```python
from build123d import *

# Parameters (mm, degrees)
SKETCH1_R           = 15.6
SKETCH1_R_2         = 14.3
BOSS_EXTRUDE1_DEPTH = 22
SKETCH2_R           = 18.1
SKETCH2_R_2         = 14.3
BOSS_EXTRUDE2_DEPTH = 3.5
FILLET1_R           = 1
CUT_EXTRUDE1_DEPTH  = 26.5


with BuildPart() as part:
    # Sketch1 → Boss-Extrude1 (new body)
    with BuildSketch(Plane(origin=(0, 0, 0), x_dir=(1, 0, 0), z_dir=(0, 1, 0))):
        Circle(SKETCH1_R)
        Circle(SKETCH1_R_2, mode=Mode.SUBTRACT)
    extrude(amount=BOSS_EXTRUDE1_DEPTH)

    # Sketch2 → Boss-Extrude2 (add)
    with BuildSketch(Plane(origin=(0, 22, 0), x_dir=(1, 0, 0), z_dir=(0, 1, 0))):
        Circle(SKETCH2_R)
        Circle(SKETCH2_R_2, mode=Mode.SUBTRACT)
    extrude(amount=BOSS_EXTRUDE2_DEPTH)

    # Fillet1
    fillet1_edges = [part.edges().sort_by_distance(p)[0] for p in [
        (-15.6, 22, 0),
    ]]
    fillet(fillet1_edges, radius=FILLET1_R)

    # Sketch3 → Cut-Extrude1 (cut, through all)
    with BuildSketch(Plane(origin=(0, 25.5, 0), x_dir=(1, 0, 0), z_dir=(0, 1, 0))):
        Polygon((0, 0), (-1.75, -18.1), (1.75, -18.1), align=None)
    extrude(amount=-CUT_EXTRUDE1_DEPTH, mode=Mode.SUBTRACT)


solid = part.part
```
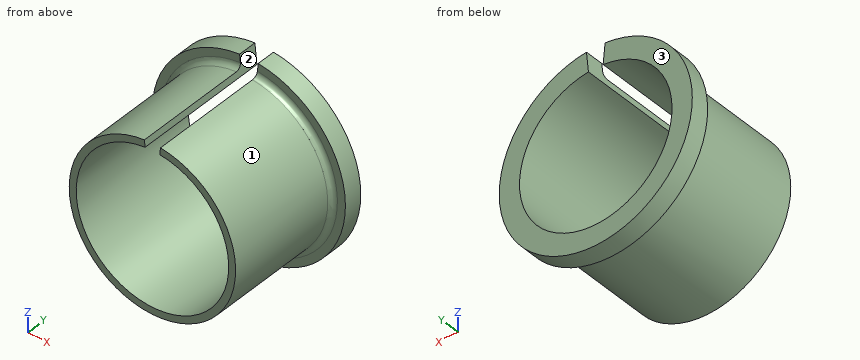
Verification items for the finished model (mm, model axes). Face numbers are marked on the shaded views. Round coordinates to 2 decimals unless told otherwise and drop trailing zeros. Write each loop counter-clockwise with the first axis right and the second up, starting at its lowest first coordinate (ties: lowest second). Pieces come first, ordered by that corner, then holes.
1. Section check D-D on y = 9.5. Enter the section's corners in (x, z), plus the area to 3 significant figures.
2. Scan lines: L1, parallel to X at y = 11.25, z = 0; L2, parallel to Z at x = 0, y = 11.5; L3, parallel to Y at x = -9.5, z = -14. Record each from-to range of solid material in increasing order.
3. Section check C-C on y = 22.75. Enter the section's corners in (x, z).
4. Draft check along X on the marked faces 1, 2 and 3. Enter one of: +X half, -X half, draft (parallel to the pull), parting line (faces both ways), or undercut.
5. Section check B-B on x = 0. Enter the section's corners in (y, z), plus the area to 3 significant figures.
6. Gauge pin test, flat ends, axial feed: P1, Ø12, axis at x = 7.5, y = 17.5, coming from the +Z side; P2, Ø12, axis at x = -6.5, y = 12.5, coming from the +Z side; P3, Ø2, axis at x = -10.5, y = 14, coming from the +Z side. Record the tip position at first contact, or that the pin passes through.
7. Section check A-A on z = 0. Enter the section's corners in (x, y).
Answer:
1. outline: (-1.5, 15.53) arc R15.6 ccw (long way) to (1.5, 15.53) - (1.38, 14.23) arc R14.3 cw (long way) to (-1.38, 14.23) - close
1. area: 118 mm2
2. L1: x = -15.6 to -14.3, 14.3 to 15.6
2. L2: z = -15.6 to -14.3
2. L3: y = 22 to 25.5
3. outline: (-1.74, 18.02) arc R18.1 ccw (long way) to (1.74, 18.02) - (1.38, 14.23) arc R14.3 cw (long way) to (-1.38, 14.23) - close
4. face 1: parting line
4. face 2: undercut
4. face 3: draft
5. outline: (0, -15.6) - (21, -15.6) arc R1 cw to (22, -16.6) - (22, -18.1) - (25.5, -18.1) - (25.5, -14.3) - (0, -14.3) - close
5. area: 42.1 mm2
6. P1: stops at z = 17.75
6. P2: stops at z = 15.53
6. P3: stops at z = 12.37
7. outline: (-18.1, 22) - (-16.6, 22) arc R1 cw to (-15.6, 21) - (-15.6, 0) - (-14.3, 0) - (-14.3, 25.5) - (-18.1, 25.5) - close; (14.3, 0) - (15.6, 0) - (15.6, 21) arc R1 cw to (16.6, 22) - (18.1, 22) - (18.1, 25.5) - (14.3, 25.5) - close
